from build123d import *

# Parameters (mm, degrees)
SKETCH4_R           = 12.7
SKETCH4_R_2         = 1.778
SKETCH4_R_3         = 2.38125
SKETCH4_R_4         = 1.75
SKETCH4_R_5         = 6
BOSS_EXTRUDE1_DEPTH = 4.572


with BuildPart() as part:
    # Sketch4 → Boss-Extrude1 (new body)
    with BuildSketch(Plane(origin=(0, 0, 0), x_dir=(0, 0, -1), z_dir=(1, 0, 0))):
        with BuildLine():
            Line((-278.598048041, 44.43052094), (-224.024344082, 27.750173837))
            ThreePointArc((-224.024344082, 27.750173837), (-213.286752868, 29.595855882), (-208.38308557, 39.325010744))
            Line((-208.38308557, 39.325010744), (-208.38308557, 191.588495768))
            ThreePointArc((-208.38308557, 191.588495768), (-208.8426278, 194.19468926), (-210.165826914, 196.486537353))
            Line((-210.165826914, 196.486537353), (-230.07024685, 220.207701322))
            ThreePointArc((-230.07024685, 220.207701322), (-232.251003102, 221.881054448), (-234.934629064, 222.476))
            Line((-234.934629064, 222.476), (-250.119258716, 222.476))
            Line((-250.119258716, 222.476), (-259.069094553, 226.862369804))
            ThreePointArc((-259.069094553, 226.862369804), (-260.42931468, 227.346249494), (-261.863679558, 227.510370624))
            Line((-261.863679558, 227.510370624), (-290.181258716, 227.510370624))
            ThreePointArc((-290.181258716, 227.510370624), (-294.671386777, 225.650498684), (-296.531258716, 221.160370624))
            Line((-296.531258716, 221.160370624), (-296.531258716, 68.663949573))
            ThreePointArc((-296.531258716, 68.663949573), (-296.13893545, 66.810982655), (-295.029296163, 65.276021876))
            ThreePointArc((-295.029296163, 65.276021876), (-276.979257712, 64.380634873), (-281.39899141, 46.857177452))
            ThreePointArc((-281.39899141, 46.857177452), (-280.255414168, 45.347331423), (-278.598048041, 44.43052094))
        make_face()
        with Locations((-229.557259723, 141.660587995)):
            Circle(SKETCH4_R, mode=Mode.SUBTRACT)
        with Locations((-221.371258716, 36.430370624)):
            Circle(SKETCH4_R_2, mode=Mode.SUBTRACT)
        with Locations((-243.629318942, 168.931188955)):
            Circle(SKETCH4_R_3, mode=Mode.SUBTRACT)
        with Locations((-280.371258716, 125.430370624)):
            Circle(SKETCH4_R_2, mode=Mode.SUBTRACT)
        with Locations((-286.371258716, 162.430370624)):
            Circle(SKETCH4_R_2, mode=Mode.SUBTRACT)
        with Locations((-279.132211518, 191.06840303)):
            Circle(SKETCH4_R_4, mode=Mode.SUBTRACT)
        with Locations((-255.799163122, 206.546414937)):
            Circle(SKETCH4_R_4, mode=Mode.SUBTRACT)
        with Locations((-263.872577413, 193.390808463)):
            Circle(SKETCH4_R_5, mode=Mode.SUBTRACT)
        with Locations((-290.871258716, 222.430370624)):
            Circle(SKETCH4_R_2, mode=Mode.SUBTRACT)
        with Locations((-234.371258716, 217.430370624)):
            Circle(SKETCH4_R_2, mode=Mode.SUBTRACT)
        with Locations((-222.371258716, 159.430370624)):
            Circle(SKETCH4_R_2, mode=Mode.SUBTRACT)
        with Locations((-265.366688027, 145.789251152)):
            Circle(SKETCH4_R_3, mode=Mode.SUBTRACT)
        with Locations((-240.13308557, 87.518200818)):
            Circle(SKETCH4_R_3, mode=Mode.SUBTRACT)
    extrude(amount=-BOSS_EXTRUDE1_DEPTH)


solid = part.part
Can you work these out from the model? Positions are in its coordinate system, mm. A direction names the side the tool comes from. Coordinates: 2 decimals unless noted, no trailing zeros. Order: outer loops, then holes, each group sorted by start corner. A loop starts at its lowest first (then second) coordinate and runs counter-clockwise, first axis right, second up. Notation, with made-up numbers: (-5.5, 12) - (9.5, 12) arc R27 cw to (9.5, 47) - close; hole circle Ø9 at (52, -3.5). An arc over 180 degrees is marked (long way). Answer as a JSON object with one key per item and string values. Group by question number.
Q1. On a 3-axis mill with a long thin cutter (end or side, diameter ignored), from which of +Z, -Z, +X, -X, +Y, -Y can I reach the whole of each face in a straight line? I mean faces 5 (the face through (-2, 227.51, 276)), 6 (the face through (-2, 222.476, 242)). Say none if no direction works.
Q2. Will these pins go through, and if not, where does the flat tip stop? P1, Ø3, axis at y = 36.43, z = 221.37, coming from the +X side; P2, Ø1, axis at x = -0.5, z = 285, coming from the -Y side.
Q3. I need wall thicknesses on line 1 (Y direction, x = -0.45, z = 235); line 2 (Z direction, x = -1.4, y = 190.5); line 3 (Y direction, x = -3.4, z = 267.5). Which ranges of each line are inside material? Lowest first, please. Write a range as from..to.
Q4. Imagine slicing it at D-D (z = 252). Please give me the cut outline in (x, y), and give its area (3 significant figures).
Q5. Imagine slicing it at A-A (y = 150). Please give me the cut outline in (x, z).
Q6. Imagine slicing it at C-C (z = 227). Please give me the cut outline in (x, y).
Q7. Imagine slicing it at B-B (x = -0.85). Give the number of separate pieces and of enclosed holes in the cut face, and give its area (3 significant figures).
Q8. We'd pull the mould along Z, two halves only. Please class faces 1 (the face through (0, 129, 253)), 2 (the face through (-2.254, 215.853, 233.551)), 3 (the face through (-2, 146, 296.531)), 4 (the face through (-2.254, 157.695, 222.757)): +Z half, -Z half, draft (parallel to the pull), parting line (faces both ways), or undercut.
Determined:
{
 "1": {"face 5": "+Z, -Z, +X, -X, +Y", "face 6": "-Z, +X, -X, +Y"},
 "2": {"P1": "passes through", "P2": "stops at y = 68.96"},
 "3": {"line 1": "y = 31.1..130.19, 153.14..215.77, 219.09..222.48", "line 2": "z = 208.38..258.61, 269.13..277.48, 280.79..296.53", "line 3": "y = 41.04..144.73, 146.85..188.61, 198.17..227.51"},
 "4": {"outline": "(-4.57, 36.3) - (0, 36.3) - (0, 223.4) - (-4.57, 223.4) - close", "area": "855 mm2"},
 "5": {"outline": "(-4.57, 208.38) - (0, 208.38) - (0, 219.98) - (-4.57, 219.98) - close; (-4.57, 239.14) - (0, 239.14) - (0, 296.53) - (-4.57, 296.53) - close"},
 "6": {"outline": "(-4.57, 28.66) - (0, 28.66) - (0, 129.22) - (-4.57, 129.22) - close; (-4.57, 154.1) - (0, 154.1) - (0, 216.55) - (-4.57, 216.55) - close"},
 "7": {"separate pieces": "1", "enclosed holes": "13", "area": "15,000 mm2"},
 "8": {"face 1": "draft", "face 2": "undercut", "face 3": "+Z half", "face 4": "undercut"}
}
